Source: CAD feature listing. Evaluate the final solid. Frame: model axes, mm. A direction names the side the tool comes from. Round coordinates to 2 decimals unless told otherwise and drop trailing zeros. Write each loop counter-clockwise with the first axis right and the second up, starting at its lowest first coordinate (ties: lowest second). Pieces come first, ordered by that corner, then holes. Notation, with made-up numbers: M 78.5,9.25 L 136.5,9.25 A22 cw 136.5,28.25 Z; hole C 36.5,-16 d7. An arc over 180 degrees is marked long. Use a Markdown table: item, result.
```python
from build123d import *

# Parameters (mm, degrees)
CROQUIS1_R              = 20
SALIENTE_EXTRUIR1_DEPTH = 7.5
CROQUIS2_R              = 7.5
SALIENTE_EXTRUIR2_DEPTH = 10
CORTAR_EXTRUIR1_DEPTH   = 10
CORTAR_EXTRUIR2_DEPTH   = 3
CORTAR_EXTRUIR3_DEPTH   = 10
CROQUIS8_R              = 1.875
CORTAR_EXTRUIR4_DEPTH   = 3
CROQUIS9_R              = 1.5
CORTAR_EXTRUIR5_DEPTH   = 10
CROQUIS10_R             = 2
CORTAR_EXTRUIR7_DEPTH   = 1


with BuildPart() as part:
    # Croquis1 → Saliente-Extruir1 (new body)
    with BuildSketch(Plane(origin=(0, 0, 0), x_dir=(1, 0, 0), z_dir=(0, 1, 0))):
        Circle(CROQUIS1_R)
    extrude(amount=SALIENTE_EXTRUIR1_DEPTH)

    # Croquis2 → Saliente-Extruir2 (add)
    with BuildSketch(Plane(origin=(0, 7.5, 0), x_dir=(1, 0, 0), z_dir=(0, 1, 0))):
        Circle(CROQUIS2_R)
    extrude(amount=SALIENTE_EXTRUIR2_DEPTH)

    # Croquis5 → Cortar-Extruir1 (cut)
    with BuildSketch(Plane(origin=(0, 17.5, 0), x_dir=(1, 0, 0), z_dir=(0, 1, 0))):
        with BuildLine():
            Line((-5, 5.590169944), (5, 5.590169944))
            ThreePointArc((5, 5.590169944), (0, 7.5), (-5, 5.590169944))
        make_face()
    extrude(amount=-CORTAR_EXTRUIR1_DEPTH, mode=Mode.SUBTRACT)

    # Croquis6 → Cortar-Extruir2 (cut)
    with BuildSketch(Plane(origin=(0, 0, -5.590169944), x_dir=(-1, 0, 0), z_dir=(0, 0, -1))):
        Polygon((0, 8.458548116), (3.5, 10.479274058), (3.5, 14.520725942), (0, 16.541451884), (-3.5, 14.520725942), (-3.5, 10.479274058), align=None)
    extrude(amount=-CORTAR_EXTRUIR2_DEPTH, mode=Mode.SUBTRACT)

    # Croquis7 → Cortar-Extruir3 (cut)
    with BuildSketch(Plane(origin=(0, 17.5, 0), x_dir=(1, 0, 0), z_dir=(0, 1, 0))):
        with BuildLine():
            Line((-1.322875656, 1.5), (1.322875656, 1.5))
            ThreePointArc((1.322875656, 1.5), (0, -2), (-1.322875656, 1.5))
        make_face()
    extrude(amount=-CORTAR_EXTRUIR3_DEPTH, mode=Mode.SUBTRACT)

    # Croquis8 → Cortar-Extruir4 (cut)
    with BuildSketch(Plane(origin=(0, 0, -2.590169944), x_dir=(-1, 0, 0), z_dir=(0, 0, -1))):
        with Locations((0, 12.5)):
            Circle(CROQUIS8_R)
    extrude(amount=-CORTAR_EXTRUIR4_DEPTH, mode=Mode.SUBTRACT)

    # Croquis9 → Cortar-Extruir5 (cut)
    with BuildSketch(Plane(origin=(0, 7.5, 0), x_dir=(1, 0, 0), z_dir=(0, 1, 0))):
        with Locations((-12.124355653, 7)):
            Circle(CROQUIS9_R)
        with Locations((12.124355653, 7)):
            Circle(CROQUIS9_R)
        with Locations((0, -14)):
            Circle(CROQUIS9_R)
    extrude(amount=-CORTAR_EXTRUIR5_DEPTH, mode=Mode.SUBTRACT)

    # Croquis10 → Cortar-Extruir7 (cut)
    with BuildSketch(Plane(origin=(0, 17.5, 0), x_dir=(1, 0, 0), z_dir=(0, 1, 0))):
        Circle(CROQUIS10_R)
    extrude(amount=-CORTAR_EXTRUIR7_DEPTH, mode=Mode.SUBTRACT)


solid = part.part
```
Q1. Section D-D on z = 0. Return loops of the section in (x, y).
Results are:
| item | result |
|---|---|
| outline | M -20,0 L 20,0 L 20,7.5 L 7.5,7.5 L 7.5,17.5 L 2,17.5 L 2,7.5 L -2,7.5 L -2,17.5 L -7.5,17.5 L -7.5,7.5 L -20,7.5 Z |
Q2. First-contact query: pin 1 Ø3 at (x, y) = (-1.5, 13.5) entering from -Z; pin 2 Ø3.5 at (x, y) = (0, 12.5) entering from +Z; pin 3 Ø6 at (x, z) = (8.5, 12.5) entering from -Y; pin 4 Ø1 at (x, z) = (-0.5, 0.5) entering from +Y. Flat tips, straight axial feed; report the tip coordinate or a pass-through.
Results are:
| item | result |
|---|---|
| pin 1 | z = -2.59 |
| pin 2 | z = 7.5 |
| pin 3 | y = 0 |
| pin 4 | y = 7.5 |
Q3. Section B-B on z = 14. Return loops of the section in (x, y).
Results are:
| item | result |
|---|---|
| outline | M -14.28,0 L -1.5,0 L -1.5,7.5 L -14.28,7.5 Z; M 1.5,0 L 14.28,0 L 14.28,7.5 L 1.5,7.5 Z |
Q4. Mould query, pull axis Y, two halves, no side actions, for faces 5 (the flat face through (0, 0, 0)), 6 (the flat face through (-1.8, 15.5, -4.1)), 7 (the flat face through (-0.1, 17.5, 2.3)). Classes: +Y half, -Y half, draft (parallel to the pull), parting line (faces both ways), or undercut.
Results are:
| item | result |
|---|---|
| face 5 | -Y half |
| face 6 | undercut |
| face 7 | +Y half |
Q5. Section A-A on y = 12.5. Return loops of the section in (x, z) (3 decimals), plus the area to 3 significant figures.
Results are:
| item | result |
|---|---|
| outline | M -5,-5.59 L -3.5,-5.59 L -3.5,-2.59 L -1.875,-2.59 L -1.875,-0.696 A2 cw long 1.875,-0.696 L 1.875,-2.59 L 3.5,-2.59 L 3.5,-5.59 L 5,-5.59 A7.5 ccw long Z |
| area | 127 mm^2 |
Q6. Line query: L1, parallel to X at y = 12, z = 0; L2, parallel to X at y = 4.5, z = -7 (3 decimals); L3, parallel to Z at x = 0, y = 2.25. Output: solid intervals per line, ascending.
Results are:
| item | result |
|---|---|
| L1 | -7.5 to -2, 2 to 7.5 |
| L2 | -18.735 to -13.624, -10.624 to 10.624, 13.624 to 18.735 |
| L3 | -20 to 12.5, 15.5 to 20 |
Q7. Reachability of faces 1 (the cylindrical face through (13.5, 3.8, -6.4)), 2 (the flat face through (-2, 16, -5.59)), 3 (the flat face through (0, 7.5, 0)), 4 (the flat face through (3.5, 13, -4)) from +Z, -Z, +X, -X, +Y, -Y: full face, straight path, thin tool, end or side. Return the list, or none.
Results are:
| item | result |
|---|---|
| face 1 | +Y, -Y |
| face 2 | -Z, +X, -X, +Y |
| face 3 | +Y |
| face 4 | -Z |
Q8. Section C-C on x = 3. Return loops of the section in (y, z).
Results are:
| item | result |
|---|---|
| outline | M 0,-19.77 L 7.5,-19.77 L 7.5,-5.59 L 10.19,-5.59 L 10.19,-2.59 L 14.81,-2.59 L 14.81,-5.59 L 17.5,-5.59 L 17.5,6.87 L 7.5,6.87 L 7.5,19.77 L 0,19.77 Z |
